```python
from build123d import *

# Parameters (mm, degrees)
SKETCH_1_W           = 17.5
SKETCH_1_H           = 17.5
EXTRUDE_1_DEPTH      = 30
SKETCH_2_W           = 20.5
SKETCH_2_H           = 20.5
SKETCH_2_W_2         = 17.5
SKETCH_2_H_2         = 17.5
EXTRUDE_2_DEPTH      = 2
SKETCH_3_W           = 26.5
SKETCH_3_H           = 26.5
SKETCH_3_W_2         = 20.5
SKETCH_3_H_2         = 20.5
EXTRUDE_3_DEPTH      = 30
SKETCH_4_R           = 2.15
CUT_EXTRUDE_6_DEPTH  = 43.164113888
SKETCH_6_W           = 10
SKETCH_6_H           = 26.5
SKETCH_6_H_2         = 6.75
EXTRUDE_5_DEPTH      = 40
SKETCH_14_R          = 1.6
CUT_EXTRUDE_9_DEPTH  = 52.983170353
SKETCH_5_R           = 2.15
CUT_EXTRUDE_10_DEPTH = 52.983170353
SKETCH_15_W          = 17.5
SKETCH_15_H          = 17.5
CUT_EXTRUDE_12_DEPTH = 28
CUT_EXTRUDE_13_DEPTH = 28
CUT_EXTRUDE_14_DEPTH = 59.099591221
SKETCH_18_R          = 16
CUT_EXTRUDE_15_DEPTH = 10
CUT_EXTRUDE_16_DEPTH = 10
SKETCH_20_W          = 40.335449496
SKETCH_20_H          = 40
CUT_EXTRUDE_17_DEPTH = 3
EXTRUDE_START        = -40
SKETCH_21_R          = 1.5
EXTRUDE_6_DEPTH      = 40
SKETCH_22_R          = 16
CUT_EXTRUDE_18_DEPTH = 40
SKETCH_24_W          = 40
SKETCH_24_H          = 40
SKETCH_24_R          = 1.6
SKETCH_24_R_2        = 14.5
EXTRUDE_7_DEPTH      = 12.5
SKETCH_25_R          = 1.6
EXTRUDE_8_DEPTH      = 7
FILLET_1_R           = 3
FILLET_2_R           = 3
FILLET_3_R           = 3
FILLET_4_R           = 3
FILLET_5_R           = 3
FILLET_6_R           = 3
FILLET_7_R           = 3
FILLET_8_R           = 3


with BuildPart() as part:
    # 草图1 → 凸台-拉伸1 (new body)
    with BuildSketch(Plane(origin=(0, 0, 0), x_dir=(0, 0, -1), z_dir=(1, 0, 0))):
        Rectangle(SKETCH_1_W, SKETCH_1_H)
    extrude(amount=EXTRUDE_1_DEPTH)

    # 草图2 → 凸台-拉伸2 (add)
    with BuildSketch(Plane.ZY):
        Rectangle(SKETCH_2_W, SKETCH_2_H)
        Rectangle(SKETCH_2_W_2, SKETCH_2_H_2, mode=Mode.SUBTRACT)
    extrude(amount=-EXTRUDE_2_DEPTH)

    # 草图3 → 凸台-拉伸3 (add)
    with BuildSketch(Plane.ZY):
        Rectangle(SKETCH_3_W, SKETCH_3_H)
        Rectangle(SKETCH_3_W_2, SKETCH_3_H_2, mode=Mode.SUBTRACT)
    extrude(amount=-EXTRUDE_3_DEPTH)

    # 草图4 → 切除-拉伸6 (cut, through all)
    with BuildSketch(Plane(origin=(0, 13.25, 0), x_dir=(1, 0, 0), z_dir=(0, 1, 0))):
        with Locations(Location((10, 0, 0), (0, 0, 270))):
            Circle(SKETCH_4_R)
        with Locations(Location((20, 0, 0), (0, 0, 270))):
            Circle(SKETCH_4_R)
    extrude(amount=-CUT_EXTRUDE_6_DEPTH, mode=Mode.SUBTRACT)

    # 草图6 → 凸台-拉伸5 (add)
    with BuildSketch(Plane.ZY):
        with Locations((-8.25, 0)):
            Rectangle(SKETCH_6_W, SKETCH_6_H)
        with Locations((-8.25, 16.625)):
            Rectangle(SKETCH_6_W, SKETCH_6_H_2)
        with Locations((-8.25, -16.625)):
            Rectangle(SKETCH_6_W, SKETCH_6_H_2)
    extrude(amount=EXTRUDE_5_DEPTH)

    # 草图14 → 切除-拉伸9 (cut, through all)
    with BuildSketch(Plane(origin=(0, 0, -13.25), x_dir=(-1, 0, 0), z_dir=(0, 0, -1))):
        with BuildLine():
            ThreePointArc((20, 15), (5, 0), (20, -15))
            Line((20, -15), (20, 15))
        make_face()
        with BuildLine():
            Line((20, 15), (20, -15))
            ThreePointArc((20, -15), (30.606601718, -10.606601718), (35, 0))
            ThreePointArc((35, 0), (30.606601718, 10.606601718), (20, 15))
        make_face()
        with Locations((5, -15)):
            Circle(SKETCH_14_R)
        with Locations((35, -15)):
            Circle(SKETCH_14_R)
        with Locations((35, 15)):
            Circle(SKETCH_14_R)
        with Locations((5, 15)):
            Circle(SKETCH_14_R)
    extrude(amount=-CUT_EXTRUDE_9_DEPTH, mode=Mode.SUBTRACT)

    # 草图5 → 切除-拉伸10 (cut, through all)
    with BuildSketch(Plane(origin=(0, 0, -13.25), x_dir=(-1, 0, 0), z_dir=(0, 0, -1))):
        with Locations(Location((-20, 0, 0), (0, 0, 180))):
            Circle(SKETCH_5_R)
        with Locations(Location((-10, 0, 0), (0, 0, 180))):
            Circle(SKETCH_5_R)
    extrude(amount=-CUT_EXTRUDE_10_DEPTH, mode=Mode.SUBTRACT)

    # 草图15 → 切除-拉伸12 (cut)
    with BuildSketch(Plane(origin=(30, 0, 0), x_dir=(0, 0, -1), z_dir=(1, 0, 0))):
        Rectangle(SKETCH_15_W, SKETCH_15_H)
    extrude(amount=-CUT_EXTRUDE_12_DEPTH, mode=Mode.SUBTRACT)

    # 草图16 → 切除-拉伸13 (cut)
    with BuildSketch(Plane.XY.offset(-3.25)):
        Polygon((-3, 0), (-6.796133828, 7.117437609), (-6.764657472, -7.058732759), align=None)
    extrude(amount=-CUT_EXTRUDE_13_DEPTH, mode=Mode.SUBTRACT)

    # 草图17 → 切除-拉伸14 (cut, through all)
    with BuildSketch(Plane(origin=(0, 20, 0), x_dir=(1, 0, 0), z_dir=(0, 1, 0))):
        with BuildLine():
            ThreePointArc((-18.5, 8.25), (-18.939339828, 9.310660172), (-20, 9.75))
            Line((-20, 9.75), (-20, 6.75))
            ThreePointArc((-20, 6.75), (-18.939339828, 7.189339828), (-18.5, 8.25))
        make_face()
        with BuildLine():
            Line((-20, 6.75), (-20, 9.75))
            ThreePointArc((-20, 9.75), (-21.5, 8.25), (-20, 6.75))
        make_face()
    extrude(amount=-CUT_EXTRUDE_14_DEPTH, mode=Mode.SUBTRACT)

    # 草图18 → 切除-拉伸15 (cut)
    with BuildSketch(Plane.XY.offset(-3.25)):
        with Locations((-20, 0)):
            Circle(SKETCH_18_R)
    extrude(amount=-CUT_EXTRUDE_15_DEPTH, mode=Mode.SUBTRACT)

    # 草图19 → 切除-拉伸16 (cut)
    with BuildSketch(Plane.XY.offset(-3.25)):
        with BuildLine():
            Line((-4.144564342, 2.145963672), (-3, 0))
            Line((-3, 0), (-2, 0))
            Line((-2, 0), (-5.777773972, 7.329958172))
            ThreePointArc((-5.777773972, 7.329958172), (-4.73943373, 4.807818333), (-4.144564342, 2.145963672))
        make_face()
        with BuildLine():
            Line((-2, 0), (-3, 0))
            Line((-3, 0), (-4.144581476, -2.146090268))
            ThreePointArc((-4.144581476, -2.146090268), (-4.739452924, -4.807879256), (-5.777773972, -7.329958172))
            Line((-5.777773972, -7.329958172), (-2, 0))
        make_face()
    extrude(amount=-CUT_EXTRUDE_16_DEPTH, mode=Mode.SUBTRACT)

    # 草图20 → 切除-拉伸17 (cut)
    with BuildSketch(Plane.XY.offset(-3.25)):
        with Locations((-20.167724748, 0)):
            Rectangle(SKETCH_20_W, SKETCH_20_H)
    extrude(amount=-CUT_EXTRUDE_17_DEPTH, mode=Mode.SUBTRACT)

    # 草图21 → 凸台-拉伸6 (add)
    with BuildSketch(Plane.XZ.offset(20).offset(EXTRUDE_START)):
        with Locations(Location((-20, -8.25, 0), (0, 0, 90))):
            Circle(SKETCH_21_R)
    extrude(amount=EXTRUDE_6_DEPTH)

    # 草图22 → 切除-拉伸18 (cut)
    with BuildSketch(Plane.XY.offset(-6.25)):
        with Locations((-20, 0)):
            Circle(SKETCH_22_R)
    extrude(amount=-CUT_EXTRUDE_18_DEPTH, mode=Mode.SUBTRACT)

    # 草图24 → 凸台-拉伸7 (add)
    with BuildSketch(Plane.XY.offset(-6.25)):
        with Locations((-20, 0)):
            Rectangle(SKETCH_24_W, SKETCH_24_H)
        with Locations(Location((-35, 15, 0), (0, 0, 180))):
            Circle(SKETCH_24_R, mode=Mode.SUBTRACT)
        with Locations(Location((-35, -15, 0), (0, 0, 180))):
            Circle(SKETCH_24_R, mode=Mode.SUBTRACT)
        with Locations(Location((-5, -15, 0), (0, 0, 180))):
            Circle(SKETCH_24_R, mode=Mode.SUBTRACT)
        with Locations(Location((-5, 15, 0), (0, 0, 180))):
            Circle(SKETCH_24_R, mode=Mode.SUBTRACT)
        with Locations((-20, 0)):
            Circle(SKETCH_24_R_2, mode=Mode.SUBTRACT)
    extrude(amount=EXTRUDE_7_DEPTH)

    # 草图25 → 凸台-拉伸8 (add)
    with BuildSketch(Plane.XY.offset(6.25)):
        Polygon((0, 20), (-40, 20), (-40, -20), (0, -20), (0, -13.25), (0, 13.25), align=None)
        with Locations(Location((-35, -15, 0), (0, 0, 180))):
            Circle(SKETCH_25_R, mode=Mode.SUBTRACT)
        with Locations(Location((-5, -15, 0), (0, 0, 180))):
            Circle(SKETCH_25_R, mode=Mode.SUBTRACT)
        with Locations(Location((-35, 15, 0), (0, 0, 180))):
            Circle(SKETCH_25_R, mode=Mode.SUBTRACT)
        with BuildLine():
            Line((-5.777773972, 7.329958172), (-2, 0))
            Line((-2, 0), (-5.777773972, -7.329958172))
            ThreePointArc((-5.777773972, -7.329958172), (-36, 0), (-5.777773972, 7.329958172))
        make_face(mode=Mode.SUBTRACT)
        with Locations(Location((-5, 15, 0), (0, 0, 180))):
            Circle(SKETCH_25_R, mode=Mode.SUBTRACT)
    extrude(amount=EXTRUDE_8_DEPTH)

    # 圆角1
    fillet_1_edges = [part.edges().sort_by_distance(p)[0] for p in [
        (0, 20, 0),
    ]]
    fillet(fillet_1_edges, radius=FILLET_1_R)

    # 圆角2
    fillet_2_edges = [part.edges().sort_by_distance(p)[0] for p in [
        (0, 13.25, 0),
    ]]
    fillet(fillet_2_edges, radius=FILLET_2_R)

    # 圆角3
    fillet_3_edges = [part.edges().sort_by_distance(p)[0] for p in [
        (-40, 20, 0),
    ]]
    fillet(fillet_3_edges, radius=FILLET_3_R)

    # 圆角4
    fillet_4_edges = [part.edges().sort_by_distance(p)[0] for p in [
        (-40, -20, 0),
    ]]
    fillet(fillet_4_edges, radius=FILLET_4_R)

    # 圆角5
    fillet_5_edges = [part.edges().sort_by_distance(p)[0] for p in [
        (0, -20, 0),
    ]]
    fillet(fillet_5_edges, radius=FILLET_5_R)

    # 圆角6
    fillet_6_edges = [part.edges().sort_by_distance(p)[0] for p in [
        (0, -13.25, 0),
    ]]
    fillet(fillet_6_edges, radius=FILLET_6_R)

    # 圆角7
    fillet_7_edges = [part.edges().sort_by_distance(p)[0] for p in [
        (0, 16.625, -13.25),
        (-0.878679656, 19.121320344, -13.25),
        (0.878679656, 14.128679656, -13.25),
        (-40, 0, -13.25),
        (-20, 20, -13.25),
        (16.5, -13.25, -13.25),
        (-39.121320344, 19.121320344, -13.25),
        (16.5, 13.25, -13.25),
        (-20, -20, -13.25),
        (-39.121320344, -19.121320344, -13.25),
        (-0.878679656, -19.121320344, -13.25),
        (0, -16.625, -13.25),
        (0.878679656, -14.128679656, -13.25),
    ]]
    fillet(fillet_7_edges, radius=FILLET_7_R)

    # 圆角8
    fillet_8_edges = [part.edges().sort_by_distance(p)[0] for p in [
        (-20, 20, 13.25),
        (-0.878679656, 19.121320344, 13.25),
        (0, 16.625, 13.25),
        (0.878679656, 14.128679656, 13.25),
        (16.5, -13.25, 13.25),
        (-40, 0, 13.25),
        (-39.121320344, 19.121320344, 13.25),
        (16.5, 13.25, 13.25),
        (-20, -20, 13.25),
        (-39.121320344, -19.121320344, 13.25),
        (0, -16.625, 13.25),
        (-0.878679656, -19.121320344, 13.25),
        (0.878679656, -14.128679656, 13.25),
    ]]
    fillet(fillet_8_edges, radius=FILLET_8_R)


solid = part.part
```
CAD build for the part. Positions are in the model's coordinates, mm. A direction names the side the tool comes from. Round coordinates to 2 decimals unless told otherwise and drop trailing zeros. Write each loop counter-clockwise with the first axis right and the second up, starting at its lowest first coordinate (ties: lowest second). Pieces come first, ordered by that corner, then holes. Notation, with made-up numbers: (37, -26) - (62, -26) arc R19 cw to (62, -13) - close; hole circle Ø9 at (-27, -6.75). An arc over 180 degrees is marked (long way). Write item = value, one per line. Start each with the question number.
Q1. Band-saw the part on D-D (x = -12.5). Give the cut face in (y, z), then the cut area to 3 significant figures.
Q2. Band-saw the part on A-A (x = 15.5). Give the cut face in (y, z).
Q3. Band-saw the part on C-C (z = 11.75). Give the cut face in (x, y), then the cut area to 3 significant figures.
Q4. Which spindle directions (+Z, -Z, +X, -X, +Y, -Y) get a long thin tool onto all of the face, cutting with end or side? Do faces 4 (the cylindrical face through (-35.99, -0.6, 9.7)), 5 (the flat face through (16, 0, 10.25)), 6 (the cylindrical face through (-0.86, -16.63, -12.35)). Say none if no direction does.
Q5. Probe L1, parallel to Y at x = 17.5, z = -1.5; L2, parallel to Y at x = -5, z = -2; L3, parallel to X at y = 11, z = -0.25. List the from-to ranges inside material, lowest first. Write a range as from..to.
Q6. Drop flat-ended pins along their axis: pin 1 (5 mm diameter, centred on x = 20, z = 0, fed in from -Y); pin 2 (1.5 mm diameter, centred on x = 15, z = -5.5, fed in from +Y); pin 3 (1.5 mm diameter, centred on y = 14.5, z = 0, fed in from +X). Give the stop position or say it passes through.
Q7. Mould opens along Z. For faces 1 (the flat face through (-9, 10, -6.25)), 2 (the cylindrical face through (-33.82, 13.92, -0.19)), 3 (the cylindrical face through (17.9, -11.73, -0.47)) say: pulls with the +Z half, pulls with the -Z half, needs draft (parallel to the pull), parting line crosses it, or undercut.
Q8. Band-saw the part on B-B (y = -8.5). Give the cut face in (x, z), then the cut area to 3 significant figures.
Answers below:
q1.outline = (-20, -10.25) arc R3 ccw to (-17, -13.25) - (-14.13, -13.25) - (-14.13, -6.25) - (-12.41, -6.25) - (-12.41, 6.25) - (-14.13, 6.25) - (-14.13, 13.25) - (-17, 13.25) arc R3 ccw to (-20, 10.25) - close; (12.41, -6.25) - (14.13, -6.25) - (14.13, -13.25) - (17, -13.25) arc R3 ccw to (20, -10.25) - (20, 10.25) arc R3 ccw to (17, 13.25) - (14.13, 13.25) - (14.13, 6.25) - (12.41, 6.25) - close
q1.area = 346 mm2
q2.outline = (-13.25, -10.25) arc R3 ccw to (-10.25, -13.25) - (10.25, -13.25) arc R3 ccw to (13.25, -10.25) - (13.25, 10.25) arc R3 ccw to (10.25, 13.25) - (-10.25, 13.25) arc R3 ccw to (-13.25, 10.25) - close; hole (-10.25, -10.25) - (10.25, -10.25) - (10.25, 10.25) - (-10.25, 10.25) - close
q3.outline = (-39.6, -17) arc R2.6 ccw to (-37, -19.6) - (-3, -19.6) arc R2.6 ccw to (-0.4, -17) - (-0.4, -16.25) arc R3.4 cw to (3, -12.85) - (30, -12.85) - (30, 12.85) - (3, 12.85) arc R3.4 cw to (-0.4, 16.25) - (-0.4, 17) arc R2.6 ccw to (-3, 19.6) - (-37, 19.6) arc R2.6 ccw to (-39.6, 17) - close; hole circle Ø3.2 at (-35, -15); hole circle Ø3.2 at (-35, 15); hole circle Ø3.2 at (-5, -15); hole circle Ø3.2 at (-5, 15); hole (-5.78, -7.33) - (-2, 0) - (-5.78, 7.33) arc R16 ccw (long way) to start; hole circle Ø4.3 at (10, 0); hole circle Ø4.3 at (20, 0)
q3.area = 1,440 mm2
q4.face_4 = +Z
q4.face_5 = +X
q4.face_6 = -Z, +X, -Y
q5.L1 = -13.25..-10.25, 10.25..13.25
q5.L2 = -20..-16.6, -13.4..13.4, 16.6..20
q5.L3 = -40..-29.45, -10.55..7.86, 12.14..17.86, 22.14..30
q6.pin_1 = -13.25
q6.pin_2 = 13.25
q6.pin_3 = 1.34
q7.face_1 = pulls with the -Z half
q7.face_2 = needs draft
q7.face_3 = undercut
q8.outline = (-40, -10.25) arc R3 ccw to (-37, -13.25) - (-33.56, -13.25) - (-33.56, -6.25) - (-31.75, -6.25) - (-31.75, 6.25) - (-33.56, 6.25) - (-33.56, 13.25) - (-37, 13.25) arc R3 ccw to (-40, 10.25) - close; (-8.25, -6.25) - (-6.44, -6.25) - (-6.44, -13.25) - (30, -13.25) - (30, -10.25) - (2, -10.25) - (2, 10.25) - (30, 10.25) - (30, 13.25) - (-6.44, 13.25) - (-6.44, 6.25) - (-8.25, 6.25) - close
q8.area = 604 mm2
